Input: part model. Units: mm. Frame: model coordinates. Face numbers are marked on the shaded views. A direction names the side the tool comes from. Coordinates: 2 decimals unless noted, no trailing zeros. Order: outer loops, then holes, each group sorted by start corner. A loop starts at its lowest first (then second) coordinate and runs counter-clockwise, first axis right, second up. Notation, with made-up numbers: (-16.75, 24.5) -> (24.25, 24.5) arc R25 cw to (24.25, 49.5) -> close; hole circle Ø4 at (26, 24.25). An arc over 180 degrees is marked (long way). One line per item, written item: value. Start each with the question number.
from build123d import *

# Parameters (mm, degrees)
BOSS_EXTRUDE1_DEPTH                     = 38.1
SKETCH2_W                               = 88.9
SKETCH2_H                               = 20.6502
CUT_EXTRUDE1_DEPTH                      = 28.575
CBORE_FOR_M8_HEX_HEAD_BOLT2_D           = 8.4
CBORE_FOR_M8_HEX_HEAD_BOLT2_CBORE_D     = 15
CBORE_FOR_M8_HEX_HEAD_BOLT2_CBORE_DEPTH = 3
CUT_EXTRUDE4_REACH                      = 66.902
FILLET1_R                               = 9.525
CUT_EXTRUDE5_START                      = -11.760877
CUT_EXTRUDE5_DEPTH                      = 11.760877
W_0_386_DIAMETER_HOLE1_D                = 9.8044
CUT_EXTRUDE7_REACH                      = 93.785
SKETCH14_W                              = 2.032
SKETCH14_H                              = 38.1


with BuildPart() as part:
    # Sketch1 → Boss-Extrude1 (new body)
    with BuildSketch(Plane(origin=(0, 0, 0), x_dir=(1, 0, 0), z_dir=(0, 1, 0))):
        Polygon((26.936371436, -17.6911), (-26.936371436, -17.6911), (-44.45, 17.6911), (44.45, 17.6911), align=None)
    extrude(amount=BOSS_EXTRUDE1_DEPTH)

    # Sketch2 → Cut-Extrude1 (cut)
    with BuildSketch(Plane(origin=(0, 38.1, 0), x_dir=(1, 0, 0), z_dir=(0, 1, 0))):
        Rectangle(SKETCH2_W, SKETCH2_H)
    extrude(amount=-CUT_EXTRUDE1_DEPTH, mode=Mode.SUBTRACT)

    # CBORE for M8 Hex Head Bolt2 (through all)
    with Locations(Plane(origin=(0, 9.525, 0), x_dir=(1, 0, 0), z_dir=(0, 1, 0))):
        with Locations((-22.225, 0), (22.225, 0)):
            CounterBoreHole(CBORE_FOR_M8_HEX_HEAD_BOLT2_D / 2, CBORE_FOR_M8_HEX_HEAD_BOLT2_CBORE_D / 2, CBORE_FOR_M8_HEX_HEAD_BOLT2_CBORE_DEPTH)

    # Sketch9 → Cut-Extrude4 (cut, up to next)
    with BuildSketch(Plane(origin=(0, 0, 10.3251), x_dir=(-1, 0, 0), z_dir=(0, 0, -1)), mode=Mode.PRIVATE) as cut_extrude4_sk1:
        Polygon((12.7, 38.1), (22.225, 9.525), (30.582424762, 9.525), (30.582424762, 38.1), align=None)
    cut_extrude4_tool1 = extrude(cut_extrude4_sk1.sketch, amount=-CUT_EXTRUDE4_REACH, mode=Mode.PRIVATE) & part.part
    # Sketch9 → Cut-Extrude4 (cut, up to next)
    with BuildSketch(Plane(origin=(0, 0, 10.3251), x_dir=(-1, 0, 0), z_dir=(0, 0, -1)), mode=Mode.PRIVATE) as cut_extrude4_sk2:
        Polygon((-30.582424762, 9.525), (-22.225, 9.525), (-12.7, 38.1), (-30.582424762, 38.1), align=None)
    cut_extrude4_tool2 = extrude(cut_extrude4_sk2.sketch, amount=-CUT_EXTRUDE4_REACH, mode=Mode.PRIVATE) & part.part
    add(cut_extrude4_tool1.solids().sort_by_distance((-23.734333, 25.541276, 10.3251))[0], mode=Mode.SUBTRACT)
    add(cut_extrude4_tool2.solids().sort_by_distance((23.734333, 25.541276, 10.3251))[0], mode=Mode.SUBTRACT)

    # Fillet1
    fillet1_edges = [part.edges().sort_by_distance(p)[0] for p in [
        (-22.225, 9.525, 14.0081),
        (22.225, 9.525, 14.0081),
    ]]
    fillet(fillet1_edges, radius=FILLET1_R)

    # Sketch10 → Cut-Extrude5 (cut)
    with BuildSketch(Plane(origin=(0, 0, -17.6911), x_dir=(-1, 0, 0), z_dir=(0, 0, -1)).offset(CUT_EXTRUDE5_START)):
        Polygon((-40.803946674, 6.35), (-19.05, 38.1), (-44.45, 38.1), (-44.45, 0), (-40.803946674, 0), align=None)
        Polygon((44.45, 38.1), (19.05, 38.1), (40.803946674, 6.35), (40.803946674, 0), (44.45, 0), align=None)
    extrude(amount=CUT_EXTRUDE5_DEPTH, mode=Mode.SUBTRACT)

    # W (0.386) Diameter Hole1 (through all)
    with Locations(Plane.XY.offset(17.6911)):
        with Locations((0, 23.392384)):
            Hole(W_0_386_DIAMETER_HOLE1_D / 2)

    # Cut-Extrude7: up to this face of the body (flat: up to its plane)
    cut_extrude7_end = Plane(part.part.faces().sort_by_distance((-40.803946674, 3.175, -14.0081))[0])
    # Sketch14 → Cut-Extrude7 (cut, up to the picked face)
    with BuildSketch(Plane(origin=(40.803946674, 0, 0), x_dir=(0, 0, -1), z_dir=(1, 0, 0)), mode=Mode.PRIVATE) as cut_extrude7_sk1:
        with Locations((-16.6751, 19.05)):
            Rectangle(SKETCH14_W, SKETCH14_H)
    cut_extrude7_tool1 = split(extrude(cut_extrude7_sk1.sketch, amount=-CUT_EXTRUDE7_REACH, mode=Mode.PRIVATE), bisect_by=cut_extrude7_end, keep=Keep.BOTH, mode=Mode.PRIVATE)
    # Sketch14 → Cut-Extrude7 (cut, up to the picked face)
    with BuildSketch(Plane(origin=(40.803946674, 0, 0), x_dir=(0, 0, -1), z_dir=(1, 0, 0)), mode=Mode.PRIVATE) as cut_extrude7_sk2:
        with Locations((16.6751, 19.05)):
            Rectangle(SKETCH14_W, SKETCH14_H)
    cut_extrude7_tool2 = split(extrude(cut_extrude7_sk2.sketch, amount=-CUT_EXTRUDE7_REACH, mode=Mode.PRIVATE), bisect_by=cut_extrude7_end, keep=Keep.BOTH, mode=Mode.PRIVATE)
    add(cut_extrude7_tool1.solids().sort_by(Axis((40.803947, 19.05, 16.6751), (-1, 0, 0)))[0], mode=Mode.SUBTRACT)
    add(cut_extrude7_tool2.solids().sort_by(Axis((40.803947, 19.05, -16.6751), (-1, 0, 0)))[0], mode=Mode.SUBTRACT)


solid = part.part
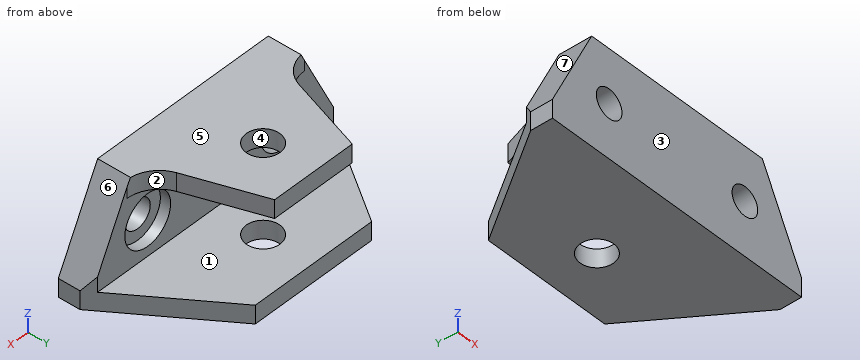
1) Section query D-D, the plane y = 8. Return the cut outline in (x, z) (3 decimals), plus the area to 3 significant figures.
2) Mould query, pull axis X, two halves, no side actions, for the marked faces 4, 5, 6 and 7. Classes: +X half, -X half, draft (parallel to the pull), parting line (faces both ways), or undercut.
3) Section query C-C, the plane z = 0. Return the cut outline in (x, y) (3 decimals), plus the area to 3 significant figures.
4) Ray query, line 1 along Z through (x, y) = (11, 17.5); line 2 along Y through (x, z) = (18, -8) (3 decimals); line 3 along Z through (x, y) = (-30.5, 10). Return the intervals inside material, ascending. Write a range as from..to.
5) Access query for the marked faces 1, 2 and 3. Directions: +Z, -Z, +X, -X, +Y, -Y. A direction counts if a zero-diameter tool reaches every point of the face in a straight line with its end or side. Return the directions, or none.
6) Pin query (flat end, axial travel): pin 1 Ø16.5 at (x, z) = (-20.5, 2) entering from +Y (3 decimals); pin 2 Ø2 at (x, y) = (-24.5, 30) entering from +Z; pin 3 Ø2 at (y, z) = (8, 1) entering from +X; pin 4 Ø8 at (x, y) = (0, 23.39) entering from -Z. Return the tip coordinate at first contact, or that it passes through.
7) Section query A-A, the plane x = 0. Return the cut outline in (y, z) (3 decimals).
8) Section query B-B, the plane y = 31.5. Return the cut outline in (x, z), plus the area to 3 significant figures.
Entries:
1. outline: (-39.673, -15.659) -> (39.673, -15.659) -> (39.673, -8.041) -> (27.942, 15.659) -> (-27.942, 15.659) -> (-39.673, -8.041) -> close; hole circle Ø15 at (-22.225, 0); hole circle Ø15 at (22.225, 0)
1. area: 1,850 mm2
2. face 4: undercut
2. face 5: draft
2. face 6: +X half
2. face 7: -X half
3. outline: (-35.693, 0) -> (-26.425, 0) -> (-26.425, 6.525) -> (-29.725, 6.525) -> (-29.725, 9.525) -> (-35.693, 9.525) -> close; (-18.025, 0) -> (18.025, 0) -> (18.025, 6.525) -> (14.725, 6.525) -> (14.725, 9.525) -> (-14.725, 9.525) -> (-14.725, 6.525) -> (-18.025, 6.525) -> close; (26.425, 0) -> (35.693, 0) -> (35.693, 9.525) -> (29.725, 9.525) -> (29.725, 6.525) -> (26.425, 6.525) -> close
3. area: 480 mm2
4. line 1: z = -15.66..-10.33, 10.33..15.66
4. line 2: y = 0..9.525
4. line 3: z = -15.66..-10.33
5. face 1: +X, -X, +Y
5. face 2: +Z, +X, +Y
5. face 3: +Z, -Z, +X, -X, -Y
6. pin 1: stops at y = 9.525
6. pin 2: stops at z = -10.33
6. pin 3: stops at x = 35.69
6. pin 4: passes through
7. outline: (0, -15.659) -> (18.49, -15.659) -> (18.49, -10.325) -> (9.525, -10.325) -> (9.525, 10.325) -> (18.49, 10.325) -> (18.49, 15.659) -> (0, 15.659) -> close; (28.295, -15.659) -> (38.1, -15.659) -> (38.1, -10.325) -> (28.295, -10.325) -> close; (28.295, 10.325) -> (38.1, 10.325) -> (38.1, 15.659) -> (28.295, 15.659) -> close
8. outline: (-23.57, -15.66) -> (23.57, -15.66) -> (23.57, -10.33) -> (-23.57, -10.33) -> close; (-14.9, 10.33) -> (14.9, 10.33) -> (14.9, 15.66) -> (-14.9, 15.66) -> close
8. area: 410 mm2
